The model under review builds one solid part; all positions refer to its coordinate system, in mm. Face numbers are marked on the shaded views. A direction names the side the tool comes from. Coordinates: 2 decimals unless noted, no trailing zeros. Loops run counter-clockwise (first coordinate to the right, second up) from the corner with the lowest first, then second, coordinate; pieces in that order, holes last. Notation, with made-up numbers: M -40,69.25 L -3,69.25 A17 cw -3,81.25 Z; hole C -29.75,-24.75 d10. An arc over 180 degrees is marked long. Use one line per item in the form item = value.
```python
from build123d import *

# Parameters (mm, degrees)
SKETCH1_R                = 4
BOSS_EXTRUDE1_DEPTH      = 28
SKETCH2_W                = 40.5
SKETCH2_H                = 38
CUT_EXTRUDE1_DEPTH       = 23
SKETCH3_R                = 9.65
CUT_EXTRUDE2_DEPTH       = 5
SKETCH8_R                = 1.15
CUT_EXTRUDE7_DEPTH       = 76.219678276
SKETCH9_R                = 2.2
CUT_EXTRUDE8_DEPTH       = 97.701654612
CUT_EXTRUDE9_DEPTH       = 3
CUT_EXTRUDE9_DEPTH_BACK  = 11
CHAMFER2_SIZE            = 3
SKETCH16_W               = 26
SKETCH16_H               = 38
CUT_EXTRUDE12_DEPTH      = 67.075411541
CUT_EXTRUDE3_START       = -5
CUT_EXTRUDE3_DEPTH       = 5
FILLET6_R                = 1.5
CUT_EXTRUDE13_START      = -5
CUT_EXTRUDE13_DEPTH      = 5
BOSS_EXTRUDE3_DEPTH      = 4.2
BOSS_EXTRUDE3_DEPTH_BACK = 4.2
SKETCH21_R               = 1.65
SKETCH15_R               = 1.7
CUT_EXTRUDE11_DEPTH      = 76.219678334
CUT_EXTRUDE14_DEPTH      = 9
FILLET1_R                = 5
FILLET2_R                = 6
FILLET4_R                = 12
CUT_EXTRUDE15_DEPTH      = 3.8
CUT_EXTRUDE18_REACH      = 77.22
SKETCH26_R               = 3.15
CUT_EXTRUDE19_START      = -12
CUT_EXTRUDE19_DEPTH      = 12
CUT_EXTRUDE20_DEPTH      = 62.824024457
CUT_EXTRUDE20_DEPTH_BACK = 4.5
SKETCH28_R               = 10
SKETCH29_W               = 23
SKETCH29_H               = 10
CUT_EXTRUDE21_DEPTH      = 8
FILLET7_R                = 8
CHAMFER1_SIZE            = 23
CHAMFER1_SIZE2           = 43.5


with BuildPart() as part:
    # Sketch1 → Boss-Extrude1 (new body)
    with BuildSketch(Plane.XY):
        with BuildLine():
            Line((-55, -23.6), (34.5, -23.6))
            Line((34.5, -23.6), (34.5, 19.4))
            Line((34.5, 19.4), (-28.5, 19.4))
            Line((-28.5, 19.4), (-28.5, 12.180409823))
            ThreePointArc((-28.5, 12.180409823), (-20.217668105, -2.285689125), (-33, -12.985083113))
            Line((-33, -12.985083113), (-36, -12.985083113))
            ThreePointArc((-36, -12.985083113), (-41.689100041, -11.672468641), (-46.228019527, -8))
            Line((-46.228019527, -8), (-55, -8))
            Line((-55, -8), (-55, -23.6))
        make_face()
        Circle(SKETCH1_R, mode=Mode.SUBTRACT)
        with BuildLine():
            Line((-23, 11.35), (-20, 11.35))
            ThreePointArc((-20, 11.35), (-18.35, 13), (-20, 14.65))
            Line((-20, 14.65), (-23, 14.65))
            ThreePointArc((-23, 14.65), (-24.65, 13), (-23, 11.35))
        make_face(mode=Mode.SUBTRACT)
        with BuildLine():
            Line((-23, -14.65), (-20, -14.65))
            ThreePointArc((-20, -14.65), (-18.35, -13), (-20, -11.35))
            Line((-20, -11.35), (-23, -11.35))
            ThreePointArc((-23, -11.35), (-24.65, -13), (-23, -14.65))
        make_face(mode=Mode.SUBTRACT)
        with BuildLine():
            Line((-46, -11.35), (-49, -11.35))
            ThreePointArc((-49, -11.35), (-50.65, -13), (-49, -14.65))
            Line((-49, -14.65), (-46, -14.65))
            ThreePointArc((-46, -14.65), (-44.35, -13), (-46, -11.35))
        make_face(mode=Mode.SUBTRACT)
    extrude(amount=BOSS_EXTRUDE1_DEPTH)

    # Sketch2 → Cut-Extrude1 (cut)
    with BuildSketch(Plane.XY.offset(28)):
        with Locations((-34.75, 0.4)):
            Rectangle(SKETCH2_W, SKETCH2_H)
    extrude(amount=-CUT_EXTRUDE1_DEPTH, mode=Mode.SUBTRACT)

    # Sketch3 → Cut-Extrude2 (cut)
    with BuildSketch(Plane.XY.offset(28)):
        Circle(SKETCH3_R)
    extrude(amount=-CUT_EXTRUDE2_DEPTH, mode=Mode.SUBTRACT)

    # Sketch8 → Cut-Extrude7 (cut, through all)
    with BuildSketch(Plane.XZ.offset(23.6)):
        with Locations(Location((3.375, 15.5, 0), (0, 0, 270))):
            Circle(SKETCH8_R)
    extrude(amount=-CUT_EXTRUDE7_DEPTH, mode=Mode.SUBTRACT)

    # Sketch9 → Cut-Extrude8 (cut, through all)
    with BuildSketch(Plane(origin=(34.5, 0, 0), x_dir=(0, 0, -1), z_dir=(1, 0, 0))):
        with Locations((-8, 13)):
            Circle(SKETCH9_R)
        with Locations((-23, 13)):
            Circle(SKETCH9_R)
    extrude(amount=-CUT_EXTRUDE8_DEPTH, mode=Mode.SUBTRACT)

    # Sketch10 → Cut-Extrude9 (cut, two sides: drawn at the far end of the back side and taken through both)
    with BuildSketch(Plane.ZY.offset(14.5).offset(-CUT_EXTRUDE9_DEPTH_BACK)):
        Polygon((5.1, 14.674315781), (5.1, 11.325684219), (8, 9.651368439), (10.9, 11.325684219), (10.9, 14.674315781), (8, 16.348631561), align=None)
        Polygon((25.9, 11.325684219), (25.9, 14.674315781), (23, 16.348631561), (20.1, 14.674315781), (20.1, 11.325684219), (23, 9.651368439), align=None)
    extrude(amount=CUT_EXTRUDE9_DEPTH + CUT_EXTRUDE9_DEPTH_BACK, mode=Mode.SUBTRACT)

    # Chamfer2
    chamfer2_edges = [part.edges().sort_by_distance(p)[0] for p in [
        (-14.5, -18.6, 16.5),
    ]]
    chamfer(chamfer2_edges, length=CHAMFER2_SIZE)

    # Sketch16 → Cut-Extrude12 (cut, through all)
    with BuildSketch(Plane.XY.offset(28)):
        with Locations((21.5, 0.4)):
            Rectangle(SKETCH16_W, SKETCH16_H)
    extrude(amount=-CUT_EXTRUDE12_DEPTH, mode=Mode.SUBTRACT)

    # Sketch4 → Cut-Extrude3 (cut)
    with BuildSketch(Plane(origin=(0, 0, 0), x_dir=(-1, 0, 0), z_dir=(0, 0, -1)).offset(CUT_EXTRUDE3_START)):
        with BuildLine():
            Line((-36.31147183, -7), (-6.642476948, -7))
            ThreePointArc((-6.642476948, -7), (9.65, 0), (-6.642476948, 7))
            Line((-6.642476948, 7), (-36.31147183, 7))
            Line((-36.31147183, 7), (-36.31147183, -7))
        make_face()
    extrude(amount=CUT_EXTRUDE3_DEPTH, mode=Mode.SUBTRACT)

    # Fillet6
    fillet6_edges = [part.edges().sort_by_distance(p)[0] for p in [
        (8.5, -18.6, 14),
    ]]
    fillet(fillet6_edges, radius=FILLET6_R)

    # Sketch17 → Cut-Extrude13 (cut)
    with BuildSketch(Plane.XY.offset(28).offset(CUT_EXTRUDE13_START)):
        with BuildLine():
            Line((0, 4), (0, 9.65))
            Line((0, 9.65), (8.5, 9.65))
            Line((8.5, 9.65), (8.5, -8.907477288))
            Line((8.5, -8.907477288), (0, -4))
            ThreePointArc((0, -4), (4, 0), (0, 4))
        make_face()
    extrude(amount=CUT_EXTRUDE13_DEPTH, mode=Mode.SUBTRACT)

    # Sketch20 → Cut-Revolve1 (revolve, cut)
    with BuildSketch(Plane.XY.offset(15.5), mode=Mode.PRIVATE) as cut_revolve1_sk:
        Polygon((3.375, -11.8), (7.375, -3.8), (3.375, -3.8), align=None)
    revolve(cut_revolve1_sk.sketch.rotate(Axis((3.375, -3.8, 15.5), (0, -1, 0)), 270), axis=Axis((3.375, -3.8, 15.5), (0, -1, 0)), mode=Mode.SUBTRACT)

    # Sketch21 → Boss-Extrude3 (add, two sides: drawn at the far end of the back side and taken through both)
    with BuildSketch(Plane.XY.offset(15.5).offset(-BOSS_EXTRUDE3_DEPTH_BACK)):
        Polygon((7.25, -8.185789452), (7.25, -18.6), (25.287941791, -18.6), align=None)
        with Locations((13.25, -15)):
            Circle(SKETCH21_R, mode=Mode.SUBTRACT)
    extrude(amount=BOSS_EXTRUDE3_DEPTH + BOSS_EXTRUDE3_DEPTH_BACK)

    # Sketch15 → Cut-Extrude11 (cut, through all)
    with BuildSketch(Plane.XZ.offset(23.6)):
        with Locations(Location((-20.625, 15, 0), (0, 0, 270))):
            Circle(SKETCH15_R)
        with Locations(Location((29.375, 15, 0), (0, 0, 270))):
            Circle(SKETCH15_R)
    extrude(amount=-CUT_EXTRUDE11_DEPTH, mode=Mode.SUBTRACT)

    # Sketch22 → Cut-Extrude14 (cut)
    with BuildSketch(Plane.XY.offset(19.7)):
        with BuildLine():
            Line((13.25, -19.5), (19.25, -19.5))
            ThreePointArc((19.25, -19.5), (23.75, -15), (19.25, -10.5))
            Line((19.25, -10.5), (13.25, -10.5))
            ThreePointArc((13.25, -10.5), (8.75, -15), (13.25, -19.5))
        make_face()
    cut_extrude14 = extrude(amount=CUT_EXTRUDE14_DEPTH, mode=Mode.SUBTRACT)

    # Mirror1: Cut-Extrude14 across plane
    add(cut_extrude14.mirror(Plane.XY.offset(15.5)), mode=Mode.SUBTRACT)

    # Fillet1
    fillet1_edges = [part.edges().sort_by_distance(p)[0] for p in [
        (-28.5, 19.4, 2.5),
    ]]
    fillet(fillet1_edges, radius=FILLET1_R)

    # Fillet2
    fillet2_edges = [part.edges().sort_by_distance(p)[0] for p in [
        (-55, -8, 2.5),
    ]]
    fillet(fillet2_edges, radius=FILLET2_R)

    # Fillet4
    fillet4_edges = [part.edges().sort_by_distance(p)[0] for p in [
        (34.5, -21.1, 28),
    ]]
    fillet(fillet4_edges, radius=FILLET4_R)

    # Sketch23 → Cut-Extrude15 (cut)
    with BuildSketch(Plane.XZ.offset(18.6)):
        Polygon((-0.775, 28.722034997), (7.525, 28.722034997), (7.525, 13.103996383), (3.375, 10.707992766), (-0.775, 13.103996383), align=None)
    extrude(amount=-CUT_EXTRUDE15_DEPTH, mode=Mode.SUBTRACT)

    # Sketch26 → Cut-Extrude18 (cut, up to next)
    with BuildSketch(Plane.XZ.offset(23.6), mode=Mode.PRIVATE) as cut_extrude18_sk1:
        with Locations(Location((3.375, 15.5, 0), (0, 0, 270))):
            Circle(SKETCH26_R)
    cut_extrude18_tool1 = extrude(cut_extrude18_sk1.sketch, amount=-CUT_EXTRUDE18_REACH, mode=Mode.PRIVATE) & part.part
    add(cut_extrude18_tool1.solids().sort_by_distance((3.375, -23.6, 15.5))[0], mode=Mode.SUBTRACT)

    # Sketch27 → Cut-Extrude19 (cut)
    with BuildSketch(Plane.XY.offset(23).offset(CUT_EXTRUDE19_START)):
        with BuildLine():
            Line((8.5, -8.907477288), (0, -4))
            ThreePointArc((0, -4), (-4, 0), (0, 4))
            Line((0, 4), (8.5, 4))
            Line((8.5, 4), (8.5, -8.907477288))
        make_face()
    extrude(amount=CUT_EXTRUDE19_DEPTH, mode=Mode.SUBTRACT)

    # Sketch28 → Cut-Extrude20 (cut, two sides: drawn at the far end of the back side and taken through both)
    with BuildSketch(Plane.XY.offset(15.5).offset(-CUT_EXTRUDE20_DEPTH_BACK)):
        with Locations((14.25, 0)):
            Circle(SKETCH28_R)
    extrude(amount=CUT_EXTRUDE20_DEPTH + CUT_EXTRUDE20_DEPTH_BACK, mode=Mode.SUBTRACT)

    # Sketch29 → Cut-Extrude21 (cut)
    with BuildSketch(Plane.ZY.offset(14.5)):
        with Locations((16.5, 14.4)):
            Rectangle(SKETCH29_W, SKETCH29_H)
    extrude(amount=-CUT_EXTRUDE21_DEPTH, mode=Mode.SUBTRACT)

    # Fillet7
    fillet7_edges = [part.edges().sort_by_distance(p)[0] for p in [
        (-14.5, 9.4, 16.5),
    ]]
    fillet(fillet7_edges, radius=FILLET7_R - 0.0001)  # a hair under: the kernel refuses the full size

    # Chamfer1
    chamfer1_edges = [part.edges().sort_by_distance(p)[0] for p in [
        (-55, -21.1, 28),
    ]]
    chamfer1_side = [part.faces().sort_by_distance(p)[0] for p in [
        (-55, -20.422699387, 12.377300613),
    ]]
    chamfer(chamfer1_edges, length=CHAMFER1_SIZE, length2=CHAMFER1_SIZE2, reference=chamfer1_side[0])


solid = part.part
```
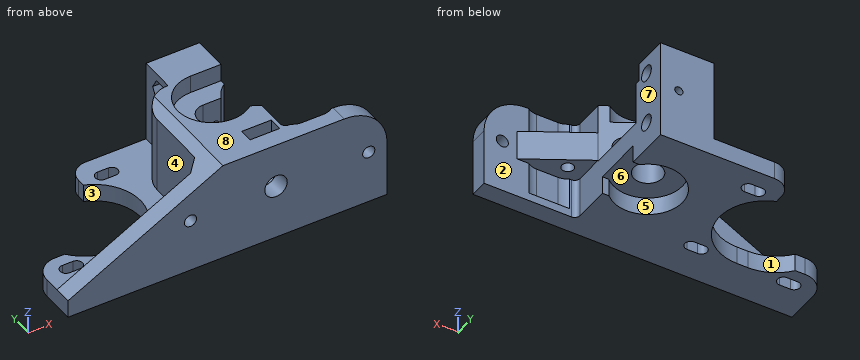
1. The part is to be moulded in two halves that separate along X. For the marked faces 6, 7 and 8, say which applies: pulls with the +X half, pulls with the -X half, needs draft (parallel to the pull), parting line crosses it, or undercut.
Response values:
face_6 = undercut
face_7 = pulls with the +X half
face_8 = needs draft
2. Insertion check: P1, Ø1.8, axis at x = 3.375, z = 15.5, coming from the +Y side; P2, Ø12, axis at y = -7.5, z = 15, coming from the -X side; P3, Ø7, axis at y = 13, z = 8, coming from the +X side; P4, Ø1, axis at y = -16, z = 7, coming from the -X side. Each pin has a flat end and moves straight along its axis. Give the tip position at first contact, or say it passes through.
Response values:
P1 = through
P2 = -14.5
P3 = 8.5
P4 = -15.4
3. Machinability: for the marked faces 1, 2, 3, 4 and 5, which of the approach directions +Z, -Z, +X, -X, +Y, -Y give a long, thin tool a straight path to every point of the face, cutting with its end or side? Answer none if there is none.
Response values:
face_1 = +Z, -Z, +Y
face_2 = +X, +Y
face_3 = +Z, -Z
face_4 = +Z, -X, +Y
face_5 = -Z
4. Add section A-A (y = 0). State the section outline as (x, z) points.
Response values:
outline = M -20.01,0 L -9.65,0 L -9.65,5 L -4,5 L -4,23 L -9.65,23 L -9.65,28 L -11.5,28 L -14.5,26.41 L -14.5,5 L -20.01,5 Z; M 4,5 L 8.5,5 L 8.5,11 L 4,11 Z
5. Wall thickness on line 1 along Y through (x, z) = (0, 2.15); line 2 along X through (y, z) = (-21.4, 15) (3 decimals); line 3 along Y through (x, z) = (0, 24.6): over which ranges is each line inside the solid? List them lowest first. Write a range as from..to.
Response values:
line_1 = -23.6..-9.65, 9.65..19.4
line_2 = -36.087..-22.325, -18.925..0.265, 6.485..27.675, 31.075..34.5
line_3 = -23.6..-18.6, -14.8..-9.65, 9.65..11.49, 14.51..19.4
